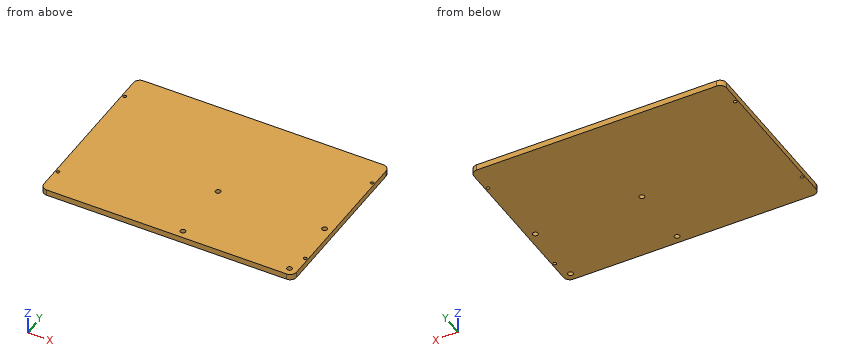
Autodesk Inventor part; units mm, degrees
ref_plane "YZ Plane" through (0, 0, 0) normal (1, 0, 0) x (0, 1, 0)
ref_plane "XZ Plane" through (0, 0, 0) normal (0, 1, 0) x (-1, 0, 0)
ref_plane "XY Plane" through (0, 0, 0) normal (0, 0, 1) x (1, 0, 0)
sketch "Sketch1" plane through (0, 0, 0) normal (0, 0, 1) x (1, 0, 0)
  line L0 (-76, 55) -> (76, 55)
  line L1 (80, 51) -> (80, -51)
  line L2 (76, -55) -> (-76, -55)
  line L3 (-80, -51) -> (-80, 51)
  arc A0 (80, 51) -> (76, 55) centre (76, 51) ccw
  arc A1 (76, -55) -> (80, -51) centre (76, -51) ccw
  arc A2 (-76, 55) -> (-80, 51) centre (-76, 51) ccw
  arc A3 (-80, -51) -> (-76, -55) centre (-76, -51) ccw
  point P0 (0, 0)
  point P1 (-80, 55)
  point P2 (80, -55)
  point P3 (80, 55)
  dimension "d0" = 160
  dimension "d1" = 110
  dimension "d2" = 55
  dimension "d3" = 80
  dimension "d4" = 4
extrude "Extrusion1" add sketch "Sketch1" along normal blind 3.75
sketch "Sketch2" plane through (0, 0, 3.75) normal (0, 0, 1) x (1, 0, 0)
  point P0 (0, 0)
  point P1 (-78.3, 38)
  point P2 (78.3, 38)
  point P3 (78.3, -38)
  point P4 (-78.3, -38)
  dimension "d7" = 156.6
  dimension "d8" = 76
  dimension "d9" = 38
  dimension "d10" = 78.3
hole "Hole1" at (-78.3, 38, 3.75) at (78.3, 38, 3.75) at (78.3, -38, 3.75) at (-78.3, -38, 3.75) direction (0, 0, -1) diameter 2.013 end through all
sketch "Sketch3" plane through (0, 0, 3.75) normal (0, 0, 1) x (1, 0, 0)
  line L0 (-76, -55) -> (76, -55)
  line L1 (80, -51) -> (80, 51)
  point P0 (0, 0)
  point P1 (7.5, -50)
  point P2 (7.5, -10)
  point P3 (75, -10)
  point P4 (75, -50)
  dimension "d18" = 40
  dimension "d19" = 67.5
  dimension "d20" = 5
  dimension "d21" = 5
hole "Hole2" at (7.5, -50, 3.75) at (7.5, -10, 3.75) at (75, -10, 3.75) at (75, -50, 3.75) direction (0, 0, -1) diameter 3.242 end through all
properties part number "sampleHolderBase_v1"
Geometry check sheet. Reference: the model listing, model coordinates, mm. Give positions to 0.01 mm unless a question says otherwise; leave off trailing zeros. Write each loop counter-clockwise with the first axis right and the second up, starting at its lowest first coordinate (ties: lowest second). Pieces come first, ordered by that corner, then holes.
1) Material ranges on L1, parallel to X at y = -38, z = 2.4; L2, parallel to Y at x = 75, z = 2.15; L3, parallel to X at y = -10, z = 2.8, recorded low to high.
2) Gauge pin test, flat end, axial feed: pin 1 (2.5 mm diameter, centred on x = 75, y = -10, fed in from +Z). Record the tip position at first contact, or that the pin passes through.
3) Section check A-A, the plane x = 7.5. Record the boundary of the cut face in (y, z), and give its area (3 significant figures).
Computed:
1. L1: x = -80 to -79.31, -77.29 to 77.29, 79.31 to 80
1. L2: y = -55 to -51.62, -48.38 to -11.62, -8.38 to 55
1. L3: x = -80 to 5.88, 9.12 to 73.38, 76.62 to 80
2. pin 1: passes through
3. outline: (-55, 0) - (-51.62, 0) - (-51.62, 3.75) - (-55, 3.75) - close; (-48.38, 0) - (-11.62, 0) - (-11.62, 3.75) - (-48.38, 3.75) - close; (-8.38, 0) - (55, 0) - (55, 3.75) - (-8.38, 3.75) - close
3. area: 388 mm2
